Source: CAD feature listing. Evaluate the final solid. Frame: model axes, mm. Coordinates: 2 decimals unless noted, no trailing zeros. Loops run counter-clockwise (first coordinate to the right, second up) from the corner with the lowest first, then second, coordinate; pieces in that order, holes last.
Item 1: Pull-direction query (Y, two-part tool) for faces 1 (the cylindrical face through (-12.534, -48.492, 0.76)), 2 (the cylindrical face through (67.53, 33.79, 0.76)), 3 (the flat face through (18, -7, 1.5)), 4 (the cylindrical face through (-9.18, -46.68, 0.74)); classes: +Y half, -Y half, draft (parallel to the pull), parting line (faces both ways), or undercut.
Item 2: Line query: probe 1 along Y at (x, z) = (9, 0.5) (3 decimals); probe 2 along X at (y, z) = (-33, 1.15) (3 decimals); probe 3 along Y at (x, z) = (28.5, 0.1) (3 decimals). Output: solid intervals per line, ascending.
Item 3: Section query C-C, the plane z = 0.75. State how many separate pieces and enclosed holes the cut face has, then the cut area to 3 significant figures.
Item 4: Section query B-B, the plane y = -12. Return the cut outline in (x, z) (3 decimals), then the cut area to 3 significant figures.
Item 5: Section query A-A, the plane x = 11.5. Return the cut outline in (y, z) (3 decimals).
Autodesk Fusion 360 part; units mm, degrees
sketch "plate-2026-01-28T23_59_03.859Z" plane through (0, 0, 0) normal (0, 0, 1) x (1, 0, 0)
  line L0 (3.025, -2.525) -> (16.025, -2.525)
  line L1 (3.025, -16.525) -> (16.025, -16.525)
  line L2 (2.525, -3.025) -> (2.525, -16.025)
  line L3 (16.525, -3.025) -> (16.525, -16.025)
  arc A0 (3.025, -2.525) -> (2.525, -3.025) centre (3.025, -3.025) ccw
  arc A1 (16.525, -3.025) -> (16.025, -2.525) centre (16.025, -3.025) ccw
  arc A2 (2.525, -16.025) -> (3.025, -16.525) centre (3.025, -16.025) ccw
  arc A3 (16.025, -16.525) -> (16.525, -16.025) centre (16.025, -16.025) ccw
  line L4 (22.075, -2.525) -> (35.075, -2.525)
  line L5 (22.075, -16.525) -> (35.075, -16.525)
  line L6 (21.575, -3.025) -> (21.575, -16.025)
  line L7 (35.575, -3.025) -> (35.575, -16.025)
  arc A4 (22.075, -2.525) -> (21.575, -3.025) centre (22.075, -3.025) ccw
  arc A5 (35.575, -3.025) -> (35.075, -2.525) centre (35.075, -3.025) ccw
  arc A6 (21.575, -16.025) -> (22.075, -16.525) centre (22.075, -16.025) ccw
  arc A7 (35.075, -16.525) -> (35.575, -16.025) centre (35.075, -16.025) ccw
  line L8 (41.125, -2.525) -> (54.125, -2.525)
  line L9 (41.125, -16.525) -> (54.125, -16.525)
  line L10 (40.625, -3.025) -> (40.625, -16.025)
  line L11 (54.625, -3.025) -> (54.625, -16.025)
  arc A8 (41.125, -2.525) -> (40.625, -3.025) centre (41.125, -3.025) ccw
  arc A9 (54.625, -3.025) -> (54.125, -2.525) centre (54.125, -3.025) ccw
  arc A10 (40.625, -16.025) -> (41.125, -16.525) centre (41.125, -16.025) ccw
  arc A11 (54.125, -16.525) -> (54.625, -16.025) centre (54.125, -16.025) ccw
  line L12 (3.025, -21.575) -> (16.025, -21.575)
  line L13 (3.025, -35.575) -> (16.025, -35.575)
  line L14 (2.525, -22.075) -> (2.525, -35.075)
  line L15 (16.525, -22.075) -> (16.525, -35.075)
  arc A12 (3.025, -21.575) -> (2.525, -22.075) centre (3.025, -22.075) ccw
  arc A13 (16.525, -22.075) -> (16.025, -21.575) centre (16.025, -22.075) ccw
  arc A14 (2.525, -35.075) -> (3.025, -35.575) centre (3.025, -35.075) ccw
  arc A15 (16.025, -35.575) -> (16.525, -35.075) centre (16.025, -35.075) ccw
  line L16 (22.075, -21.575) -> (35.075, -21.575)
  line L17 (22.075, -35.575) -> (35.075, -35.575)
  line L18 (21.575, -22.075) -> (21.575, -35.075)
  line L19 (35.575, -22.075) -> (35.575, -35.075)
  arc A16 (22.075, -21.575) -> (21.575, -22.075) centre (22.075, -22.075) ccw
  arc A17 (35.575, -22.075) -> (35.075, -21.575) centre (35.075, -22.075) ccw
  arc A18 (21.575, -35.075) -> (22.075, -35.575) centre (22.075, -35.075) ccw
  arc A19 (35.075, -35.575) -> (35.575, -35.075) centre (35.075, -35.075) ccw
  line L20 (41.125, -21.575) -> (54.125, -21.575)
  line L21 (41.125, -35.575) -> (54.125, -35.575)
  line L22 (40.625, -22.075) -> (40.625, -35.075)
  line L23 (54.625, -22.075) -> (54.625, -35.075)
  arc A20 (41.125, -21.575) -> (40.625, -22.075) centre (41.125, -22.075) ccw
  arc A21 (54.625, -22.075) -> (54.125, -21.575) centre (54.125, -22.075) ccw
  arc A22 (40.625, -35.075) -> (41.125, -35.575) centre (41.125, -35.075) ccw
  arc A23 (54.125, -35.575) -> (54.625, -35.075) centre (54.125, -35.075) ccw
sketch "Sketch2" plane through (0, 0, 0) normal (0, 0, 1) x (1, 0, 0)
sketch "Sketch3" plane through (0, 0, 0) normal (0, 0, 1) x (1, 0, 0)
  line L0 (-13.96, 35.298) -> (68.953, 35.298)
  line L1 (68.953, 35.298) -> (68.953, -49.996)
  line L2 (68.953, -49.996) -> (-13.96, -49.996)
  line L3 (-13.96, -49.996) -> (-13.96, 35.298)
  circle A0 centre (-8.96, 30.298) radius 1.7
  circle A1 centre (63.953, 30.298) radius 1.7
  circle A2 centre (-8.96, -44.996) radius 1.7
  circle A3 centre (63.953, -44.996) radius 1.7
  line L4 (18.2465, 35.298) -> (36.7465, 35.298)
  line L5 (36.7465, 35.298) -> (36.7465, 4.298)
  line L6 (36.7465, 4.298) -> (18.2465, 4.298)
  line L7 (18.2465, 4.298) -> (18.2465, 35.298)
  line L8 (2.525, -22.075) -> (2.525, -35.075)
  line L9 (3.025, -35.575) -> (16.025, -35.575)
  dimension "d1" = 82.913
  dimension "d2" = 85.294
  dimension "d5" = 3.4
  dimension "d6" = 3.4
  dimension "d7" = 3.4
  dimension "d8" = 3.4
  dimension "d9" = 5
  dimension "d10" = 5
  dimension "d11" = 5
  dimension "d12" = 5
  dimension "d13" = 5
  dimension "d14" = 5
  dimension "d15" = 5
  dimension "d16" = 5
  dimension "d17" = 18.5
  dimension "d18" = 31
  dimension "d19" = 32.2065
  dimension "d26" = 16.485
  dimension "d27" = 14.421
sketch "Sketch4" plane through (0, 0, 0) normal (0, 0, 1) x (1, 0, 0)
sketch "Sketch5" plane through (0, 0, 0) normal (0, 0, 1) x (1, 0, 0)
extrude "Extrude1" add sketch "Sketch3" along normal blind 1.5 contours L0 L1 L2 L3 L5 L6 L7
sketch "Sketch6" plane through (0, 0, 1.5) normal (0, 0, 1) x (-1, 0, 0)
  circle A0 centre (-63.953, -30.298) radius 1.7
  circle A1 centre (8.96, 44.996) radius 1.7
  circle A2 centre (-63.953, 44.996) radius 1.7
  circle A3 centre (8.96, -30.298) radius 1.7
  line L0 (-36.7465, -35.298) -> (-36.7465, -4.298)
  line L1 (-36.7465, -4.298) -> (-18.2465, -4.298)
  line L2 (-18.2465, -4.298) -> (-18.2465, -35.298)
  line L3 (-18.2465, -35.298) -> (13.96, -35.298)
  line L4 (13.96, -35.298) -> (13.96, 49.996)
  line L5 (13.96, 49.996) -> (-68.953, 49.996)
  line L6 (-68.953, 49.996) -> (-68.953, -35.298)
  line L7 (-68.953, -35.298) -> (-36.7465, -35.298)
extrude "Extrude2" cut sketch "plate-2026-01-28T23_59_03.859Z" along normal blind 1.5
fillet "Fillet1" radius 5 4 edges at (-13.96, -49.996, 0.75) (68.953, -49.996, 0.75) (-13.96, 35.298, 0.75) (68.953, 35.298, 0.75)
sketch "Sketch7" plane through (0, 0, 1.5) normal (0, 0, 1) x (-1, 0, 0)
Verdict:
1. face 1: -Y half
1. face 2: +Y half
1. face 3: draft
1. face 4: undercut
2. probe 1: y = -49.996 to -35.575, -21.575 to -16.525, -2.525 to 35.298
2. probe 2: x = -13.96 to 2.525, 16.525 to 21.575, 35.575 to 40.625, 54.625 to 68.953
2. probe 3: y = -49.996 to -35.575, -21.575 to -16.525, -2.525 to 4.298
3. separate pieces: 1
3. enclosed holes: 10
3. area: 5,270 mm2
4. outline: (-13.96, 0) - (2.525, 0) - (2.525, 1.5) - (-13.96, 1.5) - close; (16.525, 0) - (21.575, 0) - (21.575, 1.5) - (16.525, 1.5) - close; (35.575, 0) - (40.625, 0) - (40.625, 1.5) - (35.575, 1.5) - close; (54.625, 0) - (68.953, 0) - (68.953, 1.5) - (54.625, 1.5) - close
4. area: 61.4 mm2
5. outline: (-49.996, 0) - (-35.575, 0) - (-35.575, 1.5) - (-49.996, 1.5) - close; (-21.575, 0) - (-16.525, 0) - (-16.525, 1.5) - (-21.575, 1.5) - close; (-2.525, 0) - (35.298, 0) - (35.298, 1.5) - (-2.525, 1.5) - close
